Could you check a few things on this model? Use its own coordinates, in mm. A direction names the side the tool comes from. Round coordinates to 2 decimals unless told otherwise and drop trailing zeros. Write each loop counter-clockwise with the first axis right and the second up, starting at its lowest first coordinate (ties: lowest second). Pieces come first, ordered by that corner, then holes. Notation, with made-up numbers: M 26.25,6 L 43.25,6 A24 cw 43.25,21 Z; hole C 31.25,43 d8. An arc over 180 degrees is marked long. One line per item, written item: value. Start each with the question number.
(1) I want a section at B-B on y = 77. Please give me the cut outline in (x, z), and give its area (3 significant figures).
(2) I want a section at C-C on z = 26.5. Please give me the cut outline in (x, y), and give its area (3 significant figures).
(3) Which directions (+Z, -Z, +X, -X, +Y, -Y) give clear straight access to the entire face, cutting with the end or side of a thin tool? Please do faces 1 (the face through (9.86, -61.87, 50.16)), 2 (the face through (10, 50, 39.089)), 3 (the face through (10, -43.953, 26)), 4 (the face through (10, 51, 14.089)).
(4) I'm going to push flat-ended pins straight in: pin 1 Ø10 at (x, z) = (12, 20) entering from -Y; pin 2 Ø12 at (x, y) = (10, 23) entering from -Z; pin 3 Ø1.4 at (y, z) = (-49.95, 4.09) entering from -X; pin 4 Ø8 at (x, y) = (18, -1.5) entering from +Z. Where does each tip first touch, or does it pass through?
(5) Thinking about a two-plate mould opening in Z: for faces 5 (the face through (9.86, 123.48, 16.796)), 6 (the face through (10, -54, 46.589)), 7 (the face through (0, 33, 26)), which applies, released by +Z, released by -Z, zero draft, split by the parting line, or undercut?
(6) I want a section at A-A on x = 3. Please give me the cut outline in (y, z), and give its area (3 significant figures).
(7) If I drill on L1, parallel to Z at x = 15.25, y = -50; L2, parallel to Y at x = 12.25, z = 49; L3, parallel to Z at x = 16, y = 43, over which ranges is the centre line in solid material (lowest first)?
```python
from build123d import *

# Parameters (mm, degrees)
BOSS_EXTRUDE1_DEPTH = 20
SKETCH2_R           = 0.75
CUT_EXTRUDE1_DEPTH  = 140.606785953
CUT_EXTRUDE2_DEPTH  = 140.606785953
FILLET1_R           = 5
FILLET2_R           = 1
FILLET3_R           = 5
FILLET4_R           = 1
SKETCH4_W           = 19.881917645
SKETCH4_H           = 22.757656903
CUT_EXTRUDE3_DEPTH  = 140.606786098
FILLET5_R           = 5
FILLET6_R           = 1
FILLET7_R           = 5
FILLET8_R           = 1


# Some blends are built 0.0001 mm under size
with BuildPart() as part:
    # Sketch1 → Boss-Extrude1 (new body)
    with BuildSketch(Plane(origin=(0, 0, 0), x_dir=(0, 0, -1), z_dir=(1, 0, 0))):
        with BuildLine():
            Line((-39.089147287, -15.953488372), (-39.089147287, 117.046511628))
            ThreePointArc((-39.089147287, 117.046511628), (-36.453108318, 123.410472659), (-30.089147287, 126.046511628))
            Line((-30.089147287, 126.046511628), (-23.089147287, 126.046511628))
            ThreePointArc((-23.089147287, 126.046511628), (-16.725186256, 123.410472659), (-14.089147287, 117.046511628))
            Line((-14.089147287, 117.046511628), (-14.089147287, -15.953488372))
            ThreePointArc((-14.089147287, -15.953488372), (-11.746001536, -21.610342622), (-6.089147287, -23.953488372))
            Line((-6.089147287, -23.953488372), (-4.589147287, -23.953488372))
            ThreePointArc((-4.589147287, -23.953488372), (1.067706963, -26.296634123), (3.410852713, -31.953488372))
            Line((3.410852713, -31.953488372), (3.410852713, -55.953488372))
            ThreePointArc((3.410852713, -55.953488372), (1.067706963, -61.610342622), (-4.589147287, -63.953488372))
            Line((-4.589147287, -63.953488372), (-6.589147287, -63.953488372))
            Line((-6.589147287, -63.953488372), (-6.589147287, -43.953488372))
            Line((-6.589147287, -43.953488372), (-46.589147287, -43.953488372))
            Line((-46.589147287, -43.953488372), (-46.589147287, -63.953488372))
            Line((-46.589147287, -63.953488372), (-48.589147287, -63.953488372))
            ThreePointArc((-48.589147287, -63.953488372), (-54.246001536, -61.610342622), (-56.589147287, -55.953488372))
            Line((-56.589147287, -55.953488372), (-56.589147287, -31.953488372))
            ThreePointArc((-56.589147287, -31.953488372), (-54.246001536, -26.296634123), (-48.589147287, -23.953488372))
            Line((-48.589147287, -23.953488372), (-47.089147287, -23.953488372))
            ThreePointArc((-47.089147287, -23.953488372), (-41.432293037, -21.610342622), (-39.089147287, -15.953488372))
        make_face()
    extrude(amount=BOSS_EXTRUDE1_DEPTH)

    # Sketch2 → Cut-Extrude1 (cut, through all)
    with BuildSketch(Plane.ZY):
        with Locations((4.089147287, -49.953488372)):
            Circle(SKETCH2_R)
        with Locations(Location((4.089147287, -57.953488372, 0), (0, 0, 180))):
            Circle(SKETCH2_R)
        with Locations((49.089147287, -57.953488372)):
            Circle(SKETCH2_R)
        with Locations(Location((49.089147287, -49.953488372, 0), (0, 0, 180))):
            Circle(SKETCH2_R)
    extrude(amount=-CUT_EXTRUDE1_DEPTH, mode=Mode.SUBTRACT)

    # Sketch3 → Cut-Extrude2 (cut, through all)
    with BuildSketch(Plane.ZY):
        with BuildLine():
            Line((1.589147287, -43.953488372), (-3.410852713, -43.953488372))
            Line((-3.410852713, -43.953488372), (-12.995571428, -43.953488372))
            Line((-12.995571428, -43.953488372), (-12.995571428, -71.298292192))
            Line((-12.995571428, -71.298292192), (6.589147287, -71.298292192))
            Line((6.589147287, -71.298292192), (6.589147287, -63.369686859))
            ThreePointArc((6.589147287, -63.369686859), (3.053613381, -61.905220765), (1.589147287, -58.369686859))
            Line((1.589147287, -58.369686859), (1.589147287, -43.953488372))
        make_face()
        with BuildLine():
            Line((46.589147287, -63.369686859), (46.589147287, -71.298292192))
            Line((46.589147287, -71.298292192), (65.185710821, -71.298292192))
            Line((65.185710821, -71.298292192), (65.185710821, -43.953488372))
            Line((65.185710821, -43.953488372), (56.589147287, -43.953488372))
            Line((56.589147287, -43.953488372), (51.589147287, -43.953488372))
            Line((51.589147287, -43.953488372), (51.589147287, -58.369686859))
            ThreePointArc((51.589147287, -58.369686859), (50.124681193, -61.905220765), (46.589147287, -63.369686859))
        make_face()
    extrude(amount=-CUT_EXTRUDE2_DEPTH, mode=Mode.SUBTRACT)

    # Fillet1
    fillet1_edges = [part.edges().sort_by_distance(p)[0] for p in [
        (10, -43.953488372, -3.410852713),
    ]]
    fillet(fillet1_edges, radius=FILLET1_R - 0.0001)  # a hair under: the kernel refuses the full size

    # Fillet2
    fillet2_edges = [part.edges().sort_by_distance(p)[0] for p in [
        (10, -43.953488372, 1.589147287),
    ]]
    fillet(fillet2_edges, radius=FILLET2_R)

    # Fillet3
    fillet3_edges = [part.edges().sort_by_distance(p)[0] for p in [
        (10, -43.953488372, 56.589147287),
    ]]
    fillet(fillet3_edges, radius=FILLET3_R - 0.0001)  # a hair under: the kernel refuses the full size

    # Fillet4
    fillet4_edges = [part.edges().sort_by_distance(p)[0] for p in [
        (10, -43.953488372, 51.589147287),
    ]]
    fillet(fillet4_edges, radius=FILLET4_R)

    # Sketch4 → Cut-Extrude3 (cut, through all)
    with BuildSketch(Plane.ZY):
        with Locations((-8.351811536, -35.916118337)):
            Rectangle(SKETCH4_W, SKETCH4_H)
        Polygon((51.589147287, -47.294946788), (51.589147287, -22.319102336), (73.994526012, -22.319102336), (73.994526012, -45.973763973), align=None)
    extrude(amount=-CUT_EXTRUDE3_DEPTH, mode=Mode.SUBTRACT)

    # Fillet5
    # the kernel refuses this fillet: 5 mm, written as the material it takes off along each edge
    with BuildSketch(Plane(origin=(-9.996935455, -24.537289885, 1.589147287), x_dir=(0, -1, 0), z_dir=(1, 0, 0))) as fillet5_piece_1:
        with BuildLine():
            CenterArc((3.998774182, -5), FILLET5_R, 90, 66.421821522)
            ThreePointArc((-0.583801513, -3), (-0.436494933, -1.4718619), (0, 0))
            Line((0, 0), (3.998774182, 0))
        make_face()
    extrude(amount=39.99387091, mode=Mode.SUBTRACT)

    # Fillet6
    fillet6_edges = [part.edges().sort_by_distance(p)[0] for p in [
        (10, -23.953488372, 4.589147287),
    ]]
    fillet(fillet6_edges, radius=FILLET6_R)

    # Fillet7
    # the kernel refuses this fillet: 5 mm, written as the material it takes off along each edge
    with BuildSketch(Plane(origin=(29.996935455, -24.537289885, 51.589147287), x_dir=(0, -1, 0), z_dir=(-1, 0, 0))) as fillet7_piece_1:
        with BuildLine():
            CenterArc((3.998774182, -5), FILLET7_R, 90, 66.421821522)
            ThreePointArc((-0.583801513, -3), (-0.436494933, -1.4718619), (0, 0))
            Line((0, 0), (3.998774182, 0))
        make_face()
    extrude(amount=39.99387091, mode=Mode.SUBTRACT)

    # Fillet8
    fillet8_edges = [part.edges().sort_by_distance(p)[0] for p in [
        (10, -23.953488372, 48.589147287),
    ]]
    fillet(fillet8_edges, radius=FILLET8_R)


solid = part.part
```
Found:
1. outline: M 0,14.09 L 20,14.09 L 20,39.09 L 0,39.09 Z
1. area: 500 mm²
2. outline: M 0,-43.95 L 20,-43.95 L 20,126.05 L 0,126.05 Z
2. area: 3,400 mm²
3. face 1: +Z, +X, -X, -Y
3. face 2: +Z, +X, -X, +Y
3. face 3: +X, -X, -Y
3. face 4: -Z, +X, -X, +Y
4. pin 1: stops at y = -43.95
4. pin 2: stops at z = 14.09
4. pin 3: passes through
4. pin 4: stops at z = 39.09
5. face 5: released by -Z
5. face 6: undercut
5. face 7: zero draft
6. outline: M -63.37,6.59 A5 ccw -58.37,1.59 L -28.54,1.59 A5 ccw -24.06,4.37 A1 ccw -23.95,4.81 L -23.95,6.09 A8 cw -15.95,14.09 L 117.05,14.09 A9 ccw 126.05,23.09 L 126.05,30.09 A9 ccw 117.05,39.09 L -15.95,39.09 A8 cw -23.95,47.09 L -23.95,48.37 A1 ccw -24.06,48.81 A5 ccw -28.54,51.59 L -58.37,51.59 A5 ccw -63.37,46.59 L -43.95,46.59 L -43.95,6.59 Z; hole C -57.95,4.09 d1.5; hole C -57.95,49.09 d1.5; hole C -49.95,4.09 d1.5; hole C -49.95,49.09 d1.5
6. area: 4,910 mm²
7. L1: z = 1.59 to 3.34, 4.84 to 6.59, 46.59 to 48.34, 49.84 to 51.59
7. L2: y = -62.75 to -58.7, -57.21 to -50.7, -49.21 to -24.16
7. L3: z = 14.09 to 39.09
